Part model, mm, in its own coordinate system. A direction names the side the tool comes from. Round coordinates to 2 decimals unless told otherwise and drop trailing zeros. Loops run counter-clockwise (first coordinate to the right, second up) from the corner with the lowest first, then second, coordinate; pieces in that order, holes last. Notation, with made-up numbers: M -28,42.5 L 27,42.5 A25 ccw 27,55.5 Z; hole C -30,-29.75 d2. An arc over 180 degrees is marked long. Answer as CSV lines item,"result". Start each with the question number.
Item 1: Band-saw the part on B-B (y = -1). Give the cut face in (x, z).
Item 2: Band-saw the part on A-A (x = 0). Give the cut face in (y, z).
Item 3: Which spindle directions (+Z, -Z, +X, -X, +Y, -Y) get a long thin tool onto all of the face, cutting with end or side? Do faces 1 (the flat face through (-0.4, 4.1, 5)), 2 (the cylindrical face through (-3.42, -4.51, 7.46)), 3 (the flat face through (0.1, -4.3, 5)). Say none if no direction does.
Item 4: Drop flat-ended pins along their axis: pin 1 Ø1.5 at (y, z) = (-4, 4.5) entering from -X; pin 2 Ø2 at (x, z) = (3.5, 4.5) entering from -Y; pin 3 Ø2 at (x, z) = (-1.5, 4.5) entering from +Y; pin 4 Ø2 at (x, y) = (0.5, 0) entering from -Z. Give the stop position or say it passes through.
Item 5: Band-saw the part on C-C (z = 4.75). Give the cut face in (x, y).
Item 6: Mould opens along Y. For faces 4 (the cylindrical face through (0.1, -2.5, 4.9)), 5 (the flat face through (0, 2, 5)), 6 (the cylindrical face through (4.674, 2.472, 2.465)), 7 (the flat face through (-0.1, 2.2, 0)) say: pulls with the +Y half, pulls with the -Y half, needs draft (parallel to the pull), parting line crosses it, or undercut.
Item 7: Wall check: line 1 (Y direction, x = 0, z = 4.75); line 2 (Y direction, x = 0, z = 6); line 3 (Z direction, x = 1, y = 4.75). Give the ranges that are in metal, low to high.
Item 8: Band-saw the part on D-D (y = 3). Give the cut face in (x, z).
```python
from build123d import *

# Parameters (mm, degrees)
ESQUISSE1_R        = 4.9
BOSS_EXTRU_1_DEPTH = 5
ESQUISSE2_R        = 4.9
BOSS_EXTRU_2_DEPTH = 5


with BuildPart() as part:
    # Esquisse1 → Boss.-Extru.1 (new body)
    with BuildSketch(Plane.XY):
        with Locations((0, 1)):
            Circle(ESQUISSE1_R)
        with BuildLine():
            Line((-1.5, 2), (1.5, 2))
            ThreePointArc((1.5, 2), (0, -2.5), (-1.5, 2))
        make_face(mode=Mode.SUBTRACT)
    extrude(amount=BOSS_EXTRU_1_DEPTH)

    # Esquisse2 → Boss.-Extru.2 (add)
    with BuildSketch(Plane.XY.offset(5)):
        with Locations(Location((0, -1, 0), (0, 0, 168.224256014))):
            Circle(ESQUISSE2_R)
        with BuildLine():
            Line((-1.5, 2), (1.5, 2))
            ThreePointArc((1.5, 2), (0, -2.5), (-1.5, 2))
        make_face(mode=Mode.SUBTRACT)
    extrude(amount=BOSS_EXTRU_2_DEPTH)


solid = part.part
```
Answer block:
1,outline,"M -4.9,5 L -4.47,5 L -4.47,0 L -2.29,0 L -2.29,10 L -4.9,10 Z; M 2.29,0 L 4.47,0 L 4.47,5 L 4.9,5 L 4.9,10 L 2.29,10 Z"
2,outline,"M -5.9,5 L -3.9,5 L -3.9,0 L -2.5,0 L -2.5,10 L -5.9,10 Z; M 2,0 L 5.9,0 L 5.9,5 L 3.9,5 L 3.9,10 L 2,10 Z"
3,face 1,"+Z, +Y"
3,face 2,"+Z"
3,face 3,"-Z, -Y"
4,pin 1,"stops at x = -4.25"
4,pin 2,"stops at y = -5.13"
4,pin 3,"stops at y = 5.87"
4,pin 4,"passes through"
5,outline,"C 0,1 d9.8; hole M -1.5,2 A2.5 ccw long 1.5,2 Z"
6,face 4,"undercut"
6,face 5,"undercut"
6,face 6,"parting line crosses it"
6,face 7,"needs draft"
7,line 1,"y = -3.9 to -2.5, 2 to 5.9"
7,line 2,"y = -5.9 to -2.5, 2 to 3.9"
7,line 3,"z = 0 to 5"
8,outline,"M -4.47,0 L 4.47,0 L 4.47,5 L 2.83,5 L 2.83,10 L -2.83,10 L -2.83,5 L -4.47,5 Z"
